```python
from build123d import *

# Parameters (mm, degrees)
SKETCH_1_W          = 30
SKETCH_1_H          = 30
EXTRUDE_1_DEPTH     = 9
SKETCH_2_W          = 4.7
SKETCH_2_H          = 30
EXTRUDE_2_DEPTH     = 30
CUT_EXTRUDE_START   = -18.6
CUT_EXTRUDE_2_DEPTH = 18.6
SKETCH_4_R          = 4
CUT_EXTRUDE_3_DEPTH = 49.337252715
SKETCH_6_R          = 4
CUT_EXTRUDE_5_DEPTH = 37.742346142
SKETCH_7_W          = 8.2
SKETCH_7_H          = 1
EXTRUDE_3_DEPTH     = 2


# Read off the part's stored shape, not the designer's step: 切除-拉伸2
with BuildPart() as part:
    # 草图1 → 凸台-拉伸1 (new body)
    with BuildSketch(Plane.XY):
        Rectangle(SKETCH_1_W, SKETCH_1_H)
    extrude(amount=EXTRUDE_1_DEPTH)

    # 草图2 → 凸台-拉伸2 (add)
    with BuildSketch(Plane.XY.offset(9)):
        with Locations((-6.95, 0)):
            Rectangle(SKETCH_2_W, SKETCH_2_H)
        with Locations((6.95, 0)):
            Rectangle(SKETCH_2_W, SKETCH_2_H)
    extrude(amount=EXTRUDE_2_DEPTH)

    # 切除-拉伸2 outline → 切除-拉伸2 (cut)
    with BuildSketch(Plane.ZY.offset(9.3).offset(CUT_EXTRUDE_START)):
        with BuildLine():
            Line((39, 15), (24, 15))
            ThreePointArc((24, 15), (34.606601718, 10.606601718), (39, 0))
            Line((39, 0), (39, 15))
        make_face()
        with BuildLine():
            Line((39, -15), (39, 0))
            ThreePointArc((39, 0), (34.606601718, -10.606601718), (24, -15))
            Line((24, -15), (39, -15))
        make_face()
    extrude(amount=CUT_EXTRUDE_2_DEPTH, mode=Mode.SUBTRACT)

    # 草图4 → 切除-拉伸3 (cut, through all)
    with BuildSketch(Plane.ZY.offset(9.3)):
        with Locations((24, 0)):
            Circle(SKETCH_4_R)
    extrude(amount=-CUT_EXTRUDE_3_DEPTH, mode=Mode.SUBTRACT)

    # 草图6 → 切除-拉伸5 (cut, through all)
    with BuildSketch(Plane.XY.offset(9)):
        Circle(SKETCH_6_R)
    extrude(amount=-CUT_EXTRUDE_5_DEPTH, mode=Mode.SUBTRACT)

    # 草图7 → 凸台-拉伸3 (add)
    with BuildSketch(Plane(origin=(0, 0, 0), x_dir=(-1, 0, 0), z_dir=(0, 0, -1))):
        with Locations((0, 14.5)):
            Rectangle(SKETCH_7_W, SKETCH_7_H)
        with Locations((0, -14.5)):
            Rectangle(SKETCH_7_W, SKETCH_7_H)
    extrude(amount=EXTRUDE_3_DEPTH)


solid = part.part
```
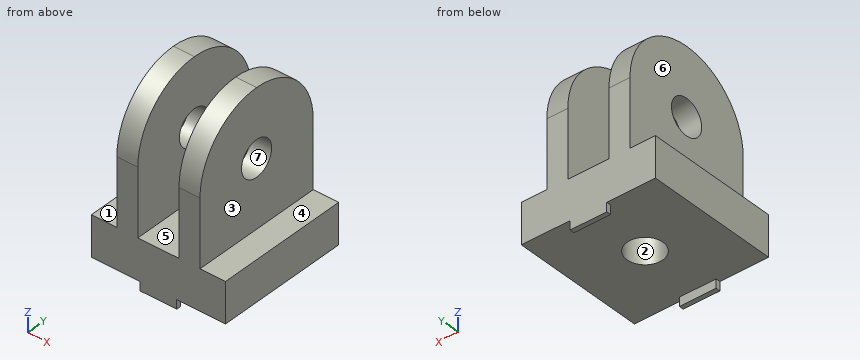
The listing builds one solid part. Answer for the finished solid, in the listing's coordinates (mm). Face numbers are marked on the shaded views. A direction names the side the tool comes from. Coordinates: 2 decimals unless noted, no trailing zeros. Write each loop counter-clockwise with the first axis right and the second up, starting at its lowest first coordinate (ties: lowest second). Pieces come first, ordered by that corner, then holes. Notation, with made-up numbers: (-1.75, 19.25) - (7.25, 19.25) arc R18 ccw to (7.25, 41.25) - close; hole circle Ø8 at (-39.5, 18.5). An arc over 180 degrees is marked (long way). One line per item, written item: value.
1) Each of these flat-tipped pins is pushed along its axis until it touches: pin 1 Ø15 at (y, z) = (-1.5, 25) entering from -X; pin 2 Ø8 at (y, z) = (-8, 35) entering from +X; pin 3 Ø0.5 at (y, z) = (14.5, -1) entering from +X; pin 4 Ø5 at (y, z) = (0, 24) entering from +X. Where does it stop, or does it pass through?
Geometry check:
pin 1: stops at x = -9.3
pin 2: stops at x = 9.3
pin 3: stops at x = 4.1
pin 4: passes through
2) A tool of negligible diameter and unlimited length cuts with its end or side. For the marked faces 4, 5, 6 and 7, from which of +Z, -Z, +X, -X, +Y, -Y can it reach the whole face along a straight path? Write none if from no direction.
Geometry check:
face 4: +Z, +X, +Y, -Y
face 5: +Z, +Y, -Y
face 6: +Z, -X, +Y, -Y
face 7: +X, -X
3) For a pull along X with two mould halves and no side action, classify the marked faces 1, 2 and 3 as pulls with the +X half, pulls with the -X half, needs draft (parallel to the pull), parting line crosses it, or undercut.
Geometry check:
face 1: needs draft
face 2: undercut
face 3: pulls with the +X half
4) Find section C-C (y = -2.75). Give the vertices of the cut face in (x, z).
Geometry check:
outline: (-15, 0) - (-2.9, 0) - (-2.9, 9) - (-4.6, 9) - (-4.6, 21.1) - (-9.3, 21.1) - (-9.3, 9) - (-15, 9) - close; (-9.3, 26.9) - (-4.6, 26.9) - (-4.6, 38.75) - (-9.3, 38.75) - close; (2.9, 0) - (15, 0) - (15, 9) - (9.3, 9) - (9.3, 21.1) - (4.6, 21.1) - (4.6, 9) - (2.9, 9) - close; (4.6, 26.9) - (9.3, 26.9) - (9.3, 38.75) - (4.6, 38.75) - close
5) Find section A-A (z = 12.5). Give the vertices of the cut face in (x, y).
Geometry check:
outline: (-9.3, -15) - (-4.6, -15) - (-4.6, 15) - (-9.3, 15) - close; (4.6, -15) - (9.3, -15) - (9.3, 15) - (4.6, 15) - close
6) Find section B-B (x = 0). Give the vertices of the cut face in (y, z), and give its area (3 significant figures).
Geometry check:
outline: (-15, -2) - (-14, -2) - (-14, 0) - (-4, 0) - (-4, 9) - (-15, 9) - close; (4, 0) - (14, 0) - (14, -2) - (15, -2) - (15, 9) - (4, 9) - close
area: 202 mm2
7) Find section D-D (z = 7). Give the vertices of the cut face in (x, y), and give its area (3 significant figures).
Geometry check:
outline: (-15, -15) - (15, -15) - (15, 15) - (-15, 15) - close; hole circle Ø8 at (0, 0)
area: 850 mm2
8) Consider line 1 along Y through (x, z) = (0, 3.75); line 2 along X through (y, z) = (7.75, 11.5); line 3 along Z through (x, y) = (-0.5, -10.5). Determine where each line is inside the solid, lowest interval first. Write a range as from..to.
Geometry check:
line 1: y = -15..-4, 4..15
line 2: x = -9.3..-4.6, 4.6..9.3
line 3: z = 0..9
